CAD build for the part. Positions are in the model's coordinates, mm. Round coordinates to 2 decimals unless told otherwise and drop trailing zeros. Loops run counter-clockwise (first coordinate to the right, second up) from the corner with the lowest first, then second, coordinate; pieces in that order, holes last. Notation, with made-up numbers: M 36.5,1 L 75.5,1 A20 ccw 75.5,17 Z; hole C -17,53.5 d7. An arc over 180 degrees is marked long. One line per item, written item: value. Start each with the question number.
from build123d import *

# Parameters (mm, degrees)
SKETCH2_W           = 8.25
SKETCH2_H           = 8.25
SKETCH2_R           = 1.65
BOSS_EXTRUDE1_DEPTH = 5


with BuildPart() as part:
    # Sketch2 → Boss-Extrude1 (new body)
    # profile 1 of 5: a face of its own
    with BuildSketch(Plane(origin=(0, 0, 0), x_dir=(1, 0, 0), z_dir=(0, 1, 0))):
        with Locations((-10, 8.875)):
            Rectangle(SKETCH2_W, SKETCH2_H)
        with Locations(Location((-10, 10, 0), (0, 0, 270))):
            Circle(SKETCH2_R, mode=Mode.SUBTRACT)
    # profile 2 of 5: a face of its own
    with BuildSketch(Plane(origin=(0, 0, 0), x_dir=(1, 0, 0), z_dir=(0, 1, 0))):
        Polygon((-22, 13), (-22, -13), (-14.125, -13), (-14.125, -4.75), (-5.875, -4.75), (-5.875, -13), (5.875, -13), (5.875, -4.75), (14.125, -4.75), (14.125, -13), (22, -13), (22, 13), (14.125, 13), (14.125, 4.75), (5.875, 4.75), (5.875, 13), (-5.875, 13), (-5.875, 4.75), (-14.125, 4.75), (-14.125, 13), align=None)
    # profile 3 of 5: a face of its own
    with BuildSketch(Plane(origin=(0, 0, 0), x_dir=(1, 0, 0), z_dir=(0, 1, 0))):
        with Locations((10, 8.875)):
            Rectangle(SKETCH2_W, SKETCH2_H)
        with Locations(Location((10, 10, 0), (0, 0, 270))):
            Circle(SKETCH2_R, mode=Mode.SUBTRACT)
    # profile 4 of 5: a face of its own
    with BuildSketch(Plane(origin=(0, 0, 0), x_dir=(1, 0, 0), z_dir=(0, 1, 0))):
        with Locations((10, -8.875)):
            Rectangle(SKETCH2_W, SKETCH2_H)
        with Locations(Location((10, -10, 0), (0, 0, 270))):
            Circle(SKETCH2_R, mode=Mode.SUBTRACT)
    # profile 5 of 5: a face of its own
    with BuildSketch(Plane(origin=(0, 0, 0), x_dir=(1, 0, 0), z_dir=(0, 1, 0))):
        with Locations((-10, -8.875)):
            Rectangle(SKETCH2_W, SKETCH2_H)
        with Locations(Location((-10, -10, 0), (0, 0, 270))):
            Circle(SKETCH2_R, mode=Mode.SUBTRACT)
    extrude(amount=-BOSS_EXTRUDE1_DEPTH)


solid = part.part
(1) Mould opens along X. For faces 1 (the flat face through (22, -2, 0)), 2 (the flat face through (0, 0, 0)), 3 (the cylindrical face through (-11.464, -2.465, 10.761)) say: pulls with the +X half, pulls with the -X half, needs draft (parallel to the pull), parting line crosses it, or undercut.
(2) Probe L1, parallel to X at y = -2.7, z = -10; L2, parallel to Z at x = -9, y = -2.2; L3, parallel to X at y = -0.4, z = 11. List the from-to ranges inside material, lowest first.
(3) Slice it at A-A, the plane x = -10. List the corners of the cut face in (y, z).
(4) Flat gauge pins, fed straight in: P1, Ø10, axis at x = 7.5, z = -7, coming from the +Y side; P2, Ø2.5, axis at x = -10, z = 10, coming from the +Y side. Where does each tip first touch, or does it go through?
(5) Slice it at B-B, the plane z = 10. List the corners of the cut face in (x, y).
(6) Slice it at C-C, the plane y = -3.15. List the corners of the cut face in (x, z).
Check result:
1. face 1: pulls with the +X half
1. face 2: needs draft
1. face 3: undercut
2. L1: x = -22 to -11.65, -8.35 to 8.35, 11.65 to 22
2. L2: z = -13 to -11.31, -8.69 to 8.69, 11.31 to 13
2. L3: x = -22 to -11.31, -8.69 to 8.69, 11.31 to 22
3. outline: M -5,-13 L 0,-13 L 0,-11.65 L -5,-11.65 Z; M -5,-8.35 L 0,-8.35 L 0,8.35 L -5,8.35 Z; M -5,11.65 L 0,11.65 L 0,13 L -5,13 Z
4. P1: stops at y = 0
4. P2: passes through
5. outline: M -22,-5 L -11.65,-5 L -11.65,0 L -22,0 Z; M -8.35,-5 L 8.35,-5 L 8.35,0 L -8.35,0 Z; M 11.65,-5 L 22,-5 L 22,0 L 11.65,0 Z
6. outline: M -22,-13 L 22,-13 L 22,13 L -22,13 Z; hole C -10,-10 d3.3; hole C -10,10 d3.3; hole C 10,-10 d3.3; hole C 10,10 d3.3
